Read the model definition and answer for the solid it produces. Units are mm, in the model's axes. A direction names the side the tool comes from. Coordinates: 2 decimals unless noted, no trailing zeros. Loops run counter-clockwise (first coordinate to the right, second up) from the corner with the lowest first, then second, coordinate; pieces in that order, holes last.
from build123d import *

# Parameters (mm, degrees)
SKETCH1_W           = 45
SKETCH1_H           = 45
BOSS_EXTRUDE1_DEPTH = 5
FILLET1_R           = 5
SKETCH4_R           = 1.925
CUT_EXTRUDE1_DEPTH  = 6
FILLET3_R           = 3
CHAMFER1_SIZE2      = 5.306388248
CHAMFER1_SIZE       = 5


with BuildPart() as part:
    # Sketch1 → Boss-Extrude1 (new body)
    with BuildSketch(Plane.XY):
        Rectangle(SKETCH1_W, SKETCH1_H)
    extrude(amount=BOSS_EXTRUDE1_DEPTH)

    # Fillet1
    fillet1_edges = [part.edges().sort_by_distance(p)[0] for p in [
        (22.5, -22.5, 2.5),
        (-22.5, -22.5, 2.5),
        (-22.5, 22.5, 2.5),
        (22.5, 22.5, 2.5),
    ]]
    fillet(fillet1_edges, radius=FILLET1_R)

    # Sketch2 → Revolve1 (revolve)
    with BuildSketch(Plane(origin=(0, 0, 0), x_dir=(1, 0, 0), z_dir=(0, 1, 0))):
        Polygon((10, 0), (5.5, 80), (0, 80), (0, 0), align=None)
    revolve(axis=Axis((0, 0, 0), (0, 0, -1)))

    # Sketch3 → Revolve2 (revolve)
    with BuildSketch(Plane(origin=(0, 0, 0), x_dir=(1, 0, 0), z_dir=(0, 1, 0))):
        with BuildLine():
            Line((0, 90), (0, 70))
            ThreePointArc((0, 70), (10, 80), (0, 90))
        make_face()
    revolve(axis=Axis((0, 0, -90), (0, 0, 1)))

    # Sketch4 → Cut-Extrude1 (cut, through all)
    with BuildSketch(Plane(origin=(0, 0, 0), x_dir=(-1, 0, 0), z_dir=(0, 0, -1))):
        with Locations((15, 15)):
            Circle(SKETCH4_R)
        with Locations((15, -15)):
            Circle(SKETCH4_R)
        with Locations((-15, -15)):
            Circle(SKETCH4_R)
        with Locations((-15, 15)):
            Circle(SKETCH4_R)
    extrude(amount=-CUT_EXTRUDE1_DEPTH, mode=Mode.SUBTRACT)

    # Fillet3
    fillet3_edges = [part.edges().sort_by_distance(p)[0] for p in [
        (-5.952011904, 0, -71.964232813),
    ]]
    fillet(fillet3_edges, radius=FILLET3_R)

    # Chamfer1
    chamfer1_edges = [part.edges().sort_by_distance(p)[0] for p in [
        (-10, 0, 0),
    ]]
    chamfer(chamfer1_edges, length=CHAMFER1_SIZE, length2=CHAMFER1_SIZE2)


solid = part.part
Item 1: Given pin 1 (10 mm diameter, centred on x = 7.5, z = -36, fed in from +Y); pin 2 (8 mm diameter, centred on y = 11, z = -31, fed in from -X); pin 3 (3 mm diameter, centred on x = 6.5, y = 2, fed in from -Z); pin 4 (6 mm diameter, centred on x = -14.5, z = -5, fed in from -Y), each flat-ended and moving along its own axis, determine where each tip first touches the part or whether it passes through.
Numbers:
pin 1: stops at y = 7.6
pin 2: stops at x = -4.39
pin 3: stops at z = -88.48
pin 4: passes through
Item 2: A cutting plane is placed at C-C on z = -14. Determine the outline of the cut face in (x, y) (1 decimal).
Numbers:
outline: circle Ø18.4 at (0, 0)
Item 3: A cutting plane is placed at B-B on z = -75. Determine the outline of the cut face in (x, y), then the cut area to 3 significant figures.
Numbers:
outline: circle Ø17.32 at (0, 0)
area: 236 mm2
Item 4: A cutting plane is placed at A-A on x = -18.5. Determine the outline of the cut face in (y, z), then the cut area to 3 significant figures.
Numbers:
outline: (-22.4, 0) - (22.4, 0) - (22.4, 5) - (-22.4, 5) - close
area: 224 mm2
Item 5: Determine the mould class of faces 1 (the face through (0, -22.5, 2)), 2 (the face through (-1.702, 7.665, -38.195)), 3 (the face through (-14.7, 16.9, 2.5)) for opening direction Y: released by +Y, released by -Y, zero draft, split by the parting line, or undercut.
Numbers:
face 1: released by -Y
face 2: split by the parting line
face 3: undercut
Item 6: Find the intervals of material crossed by line 1 along Y through (x, z) = (-15, 1) (3 decimals); line 2 along Z through (x, y) = (17.5, 2.5); line 3 along Z through (x, y) = (0.5, 12.5), in increasing order.
Numbers:
line 1: y = -22.5 to -16.925, -13.075 to 13.075, 16.925 to 22.5
line 2: z = 0 to 5
line 3: z = -2.5 to 5
Item 7: Which of the six approach directions +Z, -Z, +X, -X, +Y, -Y give full straight-line access (tool end or side, diameter ignored) to faces 4 (the face through (-21.07, -21, 2.54)), 5 (the face through (-5, 15, 0))?
Numbers:
face 4: +Z, -Z, -X, -Y
face 5: -Z
